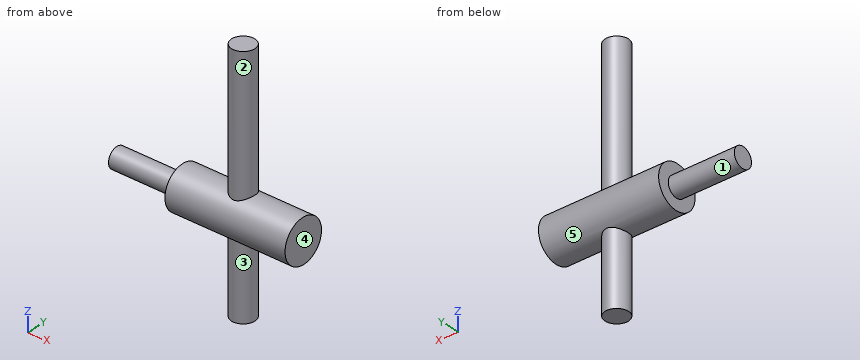
from build123d import *

# Parameters (mm, degrees)
CYLINDER001_R     = 1.65
CYLINDER001_DEPTH = 11
CYLINDER_R        = 3.5
CYLINDER_DEPTH    = 20
CYLINDER002_R     = 1.9
CYLINDER002_DEPTH = 40


with BuildPart() as cylinder001:
    # Cylinder001 → Cylinder001 (new body)
    with BuildSketch(Plane(origin=(-10, 0, 15), x_dir=(0, 0, 1), z_dir=(-1, 0, 0))):
        Circle(CYLINDER001_R)
    extrude(amount=CYLINDER001_DEPTH)


with BuildPart() as cylinder:
    # Cylinder → Cylinder (new body)
    with BuildSketch(Plane(origin=(10, 0, 15), x_dir=(0, 0, 1), z_dir=(-1, 0, 0))):
        Circle(CYLINDER_R)
    extrude(amount=CYLINDER_DEPTH)


with BuildPart() as bolt_slot:
    # Cylinder002 → Cylinder002 (new body)
    with BuildSketch(Plane.XY):
        Circle(CYLINDER002_R)
    extrude(amount=CYLINDER002_DEPTH)

    # Fusion001010002: union Cylinder001, Cylinder
    add(cylinder001.part)
    add(cylinder.part)


solid = bolt_slot.part
Geometry check sheet. Reference: the model listing, model coordinates, mm. Face numbers are marked on the shaded views. A direction names the side the tool comes from. Give positions to 0.01 mm unless a question says otherwise; leave off trailing zeros. Loops run counter-clockwise (first coordinate to the right, second up) from the corner with the lowest first, then second, coordinate; pieces in that order, holes last. Notation, with made-up numbers: (-32, -34) -> (-27, -34) arc R27 ccw to (-27, -11) -> close; hole circle Ø6 at (23, 69.5). An arc over 180 degrees is marked (long way). Answer in a Markdown table with one row per item. Add a question column.
1) Cross-section at A-A on z = 15. Record the boundary of the cut face in (x, y).
2) Gauge pin test, flat ends, axial feed: P1, Ø5, axis at x = -6.5, z = 20.5, coming from the +Y side; P2, Ø10, axis at x = 4.5, z = 32, coming from the +Y side; P3, Ø1, axis at x = 3.5, y = -0.5, coming from the +Z side. Record the tip position at first contact, or that the pin passes through.
3) Material ranges on probe 1 along X at (y, z) = (1, 12); probe 2 along Z at (x, y) = (8, 0); probe 3 along Z at (x, y) = (7, 1.5), recorded low to high. Write a range as from..to.
4) Cross-section at C-C on x = 0. Record the boundary of the cut face in (y, z), and give its area (3 significant figures).
5) Set-up check for the marked faces 1, 2, 3, 4 and 5: record each of +Z, -Z, +X, -X, +Y, -Y from which the full face is reachable in a straight line by a thin tool's end or side.
6) Cross-section at B-B on y = 0. Record the boundary of the cut face in (x, z), and give its area (3 significant figures).
7) Cross-section at D-D on x = -9. Record the boundary of the cut face in (y, z).
Outcome:
| question | item | result |
|---|---|---|
| 1 | outline | (-21, -1.65) -> (-10, -1.65) -> (-10, -3.5) -> (10, -3.5) -> (10, 3.5) -> (-10, 3.5) -> (-10, 1.65) -> (-21, 1.65) -> close |
| 2 | P1 | stops at y = 1.8 |
| 2 | P2 | stops at y = 1.9 |
| 2 | P3 | stops at z = 18.5 |
| 3 | probe 1 | x = -10..10 |
| 3 | probe 2 | z = 11.5..18.5 |
| 3 | probe 3 | z = 11.84..18.16 |
| 4 | outline | (-1.9, 0) -> (1.9, 0) -> (1.9, 12.06) arc R3.5 ccw to (1.9, 17.94) -> (1.9, 40) -> (-1.9, 40) -> (-1.9, 17.94) arc R3.5 ccw to (-1.9, 12.06) -> close |
| 4 | area | 165 mm^2 |
| 5 | face 1 | -X |
| 5 | face 2 | +Z |
| 5 | face 3 | -Z |
| 5 | face 4 | +Z, -Z, +X, +Y, -Y |
| 5 | face 5 | none |
| 6 | outline | (-21, 13.35) -> (-10, 13.35) -> (-10, 11.5) -> (-1.9, 11.5) -> (-1.9, 0) -> (1.9, 0) -> (1.9, 11.5) -> (10, 11.5) -> (10, 18.5) -> (1.9, 18.5) -> (1.9, 40) -> (-1.9, 40) -> (-1.9, 18.5) -> (-10, 18.5) -> (-10, 16.65) -> (-21, 16.65) -> close |
| 6 | area | 302 mm^2 |
| 7 | outline | circle Ø7 at (0, 15) |
